```python
from build123d import *

# Parameters (mm, degrees)
F0_R     = 19.35
F1_DEPTH = 13.2
F2_R     = 1.5
F3_DEPTH = 43.2
F4_R     = 19.35
F5_DEPTH = 13.2
F6_R     = 2


with BuildPart() as f1:
    # F0 (on Right) → F1 (new body)
    with BuildSketch(Plane.YZ):
        Circle(F0_R)
    extrude(amount=F1_DEPTH)

    # F2 (on face) → F3 (join)
    with BuildSketch(Plane.YZ.offset(13.2)):
        Circle(F2_R)
    extrude(amount=F3_DEPTH)

    # F4 (on face) → F5 (join)
    with BuildSketch(Plane.YZ.offset(56.4)):
        Circle(F4_R)
    extrude(amount=F5_DEPTH)

    # F6
    f6_edges = [f1.edges().sort_by_distance(p)[0] for p in [
        (0, -19.35, 0),
        (13.2, -19.35, 0),
        (56.4, -19.35, 0),
        (69.6, -19.35, 0),
    ]]
    fillet(f6_edges, radius=F6_R)


solid = f1.part
```
Here's how the part is built. I have some questions about the finished solid (model axes, mm). A direction names the side the tool comes from. Give positions to 0.01 mm unless a question says otherwise; leave off trailing zeros. Loops run counter-clockwise (first coordinate to the right, second up) from the corner with the lowest first, then second, coordinate; pieces in that order, holes last. Notation, with made-up numbers: M 31.5,53 L 45.5,53 A10 ccw 45.5,65 Z; hole C -23,-32 d11. An arc over 180 degrees is marked long. Use one line per item in the form item = value. Start each with the question number.
Q1. I need wall thicknesses on line 1 along X through (y, z) = (2, -9); line 2 along Z through (x, y) = (9, -7); line 3 along Z through (x, y) = (8.5, 11). Which ranges of each line are inside material? Lowest first, please.
Q2. If we section it at D-D (x = 63): Write out the boundary of the cut face in (y, z).
Q3. Will these pins go through, and if not, where does the flat tip stop? pin 1 Ø8 at (x, z) = (49.5, 3.5) entering from -Y; pin 2 Ø1 at (x, z) = (10.5, -1.5) entering from -Y; pin 3 Ø3 at (y, z) = (-6, 5.5) entering from -X; pin 4 Ø3 at (x, z) = (33, -1) entering from +Y.
Q4. Which directions (+Z, -Z, +X, -X, +Y, -Y) give clear straight access to the entire face, cutting with the end or side of a thin tool? Please do faces 1 (the cylindrical face through (62.94, -19.33, 0.85)), 2 (the cylindrical face through (34.5, -1.5, 0.07)).
Q5. If we section it at A-A (z = 0): Write out the boundary of the cut face in (x, y).
Q6. Thinking about a two-plate mould opening in X: for faces 3 (the cylindrical face through (6.54, -19.33, 0.85)), 4 (the flat face through (13.2, 4, 0)), 5 (the flat face through (69.6, 0, 0)), which applies, +X half, -X half, draft (parallel to the pull), parting line (faces both ways), or undercut?
Q7. If we section it at C-C (x = 20.5): Write out the boundary of the cut face in (y, z), then the cut area to 3 significant figures.
Taken from the geometry:
q1.line_1 = 0 to 13.2, 56.4 to 69.6
q1.line_2 = -18.04 to 18.04
q1.line_3 = -15.92 to 15.92
q2.outline = C 0,0 d38.7
q3.pin_1 = -1.5
q3.pin_2 = -19.32
q3.pin_3 = 0
q3.pin_4 = 1.5
q4.face_1 = +X, -X
q4.face_2 = none
q5.outline = M 0,-17.35 A2 ccw 2,-19.35 L 11.2,-19.35 A2 ccw 13.2,-17.35 L 13.2,-1.5 L 56.4,-1.5 L 56.4,-17.35 A2 ccw 58.4,-19.35 L 67.6,-19.35 A2 ccw 69.6,-17.35 L 69.6,17.35 A2 ccw 67.6,19.35 L 58.4,19.35 A2 ccw 56.4,17.35 L 56.4,1.5 L 13.2,1.5 L 13.2,17.35 A2 ccw 11.2,19.35 L 2,19.35 A2 ccw 0,17.35 Z
q6.face_3 = draft
q6.face_4 = undercut
q6.face_5 = +X half
q7.outline = C 0,0 d3
q7.area = 7.07 mm^2
